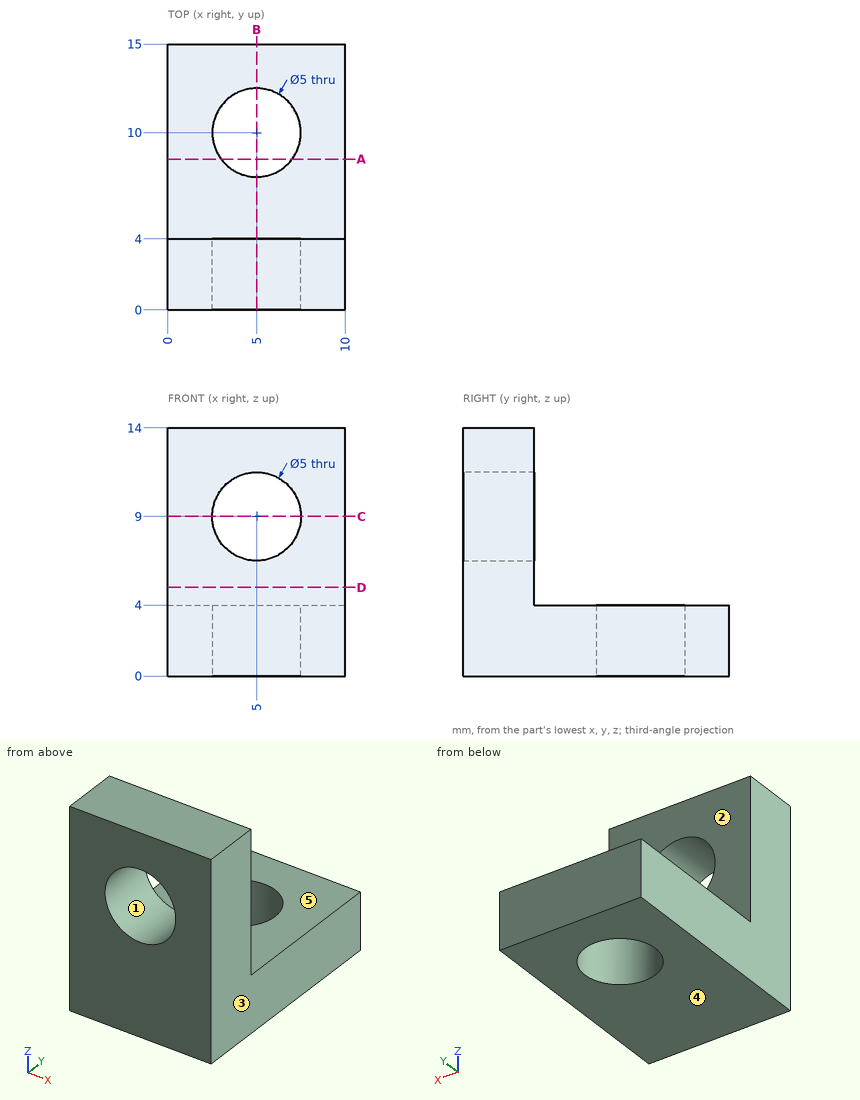
Input: dimensioned drawing with shaded views. Units: mm. Origin: part minimum x, y, z. A direction names the side the tool comes from. Coordinates: 2 decimals unless noted, no trailing zeros. Loops run counter-clockwise (first coordinate to the right, second up) from the corner with the lowest first, then second, coordinate; pieces in that order, holes last. Notation, with made-up numbers: M 50,50 L 71,50 A24 ccw 71,83 Z; hole C 28.5,-16 d1. An arc over 180 degrees is marked long. Use a Markdown table: item, result. Add a question column.
1) Line query: L1, parallel to Y at x = 5, z = 2.85; L2, parallel to Y at x = 7.5, z = 10.5. Output: solid intervals per line, ascending. Write a range as from..to.
2) Section B-B, the plane x = 5. Return the cut outline in (y, z).
3) Draft query along X for the marked faces 1, 2 and 3. Return one class per face: +X half, -X half, draft (parallel to the pull), parting line (faces both ways), or undercut.
4) Section C-C, the plane z = 9. Return the cut outline in (x, y), plus the area to 3 significant figures.
5) Section A-A, the plane y = 8.5. Return the cut outline in (x, z), plus the area to 3 significant figures.
6) Set-up query: the marked faces 4 and 5. Return all of +Z, -Z, +X, -X, +Y, -Y with unobstructed straight access to the full face (end or side cutting, diameter ignored); none if empty.
7) Pin query (flat end, axial travel): P1, Ø5, axis at x = 3, z = 11, coming from the +Y side; P2, Ø1, axis at x = 3, y = 11.5, coming from the +Z side. Return the tip coordinate at first contact, or that it passes through.
8) Section D-D, the plane z = 5. Return the cut outline in (x, y).
Answer below:
| question | item | result |
|---|---|---|
| 1 | L1 | 0..7.5, 12.5..15 |
| 1 | L2 | 0..4 |
| 2 | outline | M 0,0 L 7.5,0 L 7.5,4 L 4,4 L 4,6.5 L 0,6.5 Z; M 0,11.5 L 4,11.5 L 4,14 L 0,14 Z; M 12.5,0 L 15,0 L 15,4 L 12.5,4 Z |
| 3 | face 1 | undercut |
| 3 | face 2 | draft |
| 3 | face 3 | +X half |
| 4 | outline | M 0,0 L 2.5,0 L 2.5,4 L 0,4 Z; M 7.5,0 L 10,0 L 10,4 L 7.5,4 Z |
| 4 | area | 20.0 mm2 |
| 5 | outline | M 0,0 L 3,0 L 3,4 L 0,4 Z; M 7,0 L 10,0 L 10,4 L 7,4 Z |
| 5 | area | 24.0 mm2 |
| 6 | face 4 | -Z, +X, -X, +Y, -Y |
| 6 | face 5 | +Z, +X, -X, +Y |
| 7 | P1 | y = 4 |
| 7 | P2 | z = 4 |
| 8 | outline | M 0,0 L 10,0 L 10,4 L 0,4 Z |
